Could you check a few things on this drawing? It's one solid part, dimensions in mm from its lowest x, y, z. A direction names the side the tool comes from. Give positions to 0.01 mm unless a question says otherwise; leave off trailing zeros. Loops run counter-clockwise (first coordinate to the right, second up) from the corner with the lowest first, then second, coordinate; pieces in that order, holes last. Notation, with made-up numbers: M 66,3 L 85,3 A37 cw 85,39 Z; hole C 36.5,30 d2. An arc over 180 degrees is marked long. Answer in a Markdown table with one row per item. Add a question column.
1. Which directions (+Z, -Z, +X, -X, +Y, -Y) give clear straight access to the entire face, cutting with the end or side of a thin tool? Please do the marked faces 1 and 2.
2. If we section it at A-A on x = 20: List the corners of the cut face in (y, z) for me.
3. I need wall thicknesses on line 1 along Z through (x, y) = (22.5, 36.5); line 2 along Y through (x, z) = (19.5, 6.5); line 3 along Y through (x, z) = (12, 4). Which ranges of each line are inside material? Lowest first, please. Write a range as from..to.
4. If we section it at C-C on z = 29: List the corners of the cut face in (x, y) for me, then the cut area to 3 significant figures.
5. I'm going to push flat-ended pins straight in: pin 1 Ø2 at (x, z) = (27.5, 11.5) entering from -Y; pin 2 Ø1.5 at (x, z) = (25.5, 8) entering from +Y; pin 3 Ø8 at (x, z) = (11.5, 21) entering from -Y. Where does each tip first touch, or does it pass through?
6. If we section it at D-D on x = 34.5: List the corners of the cut face in (y, z) for me.
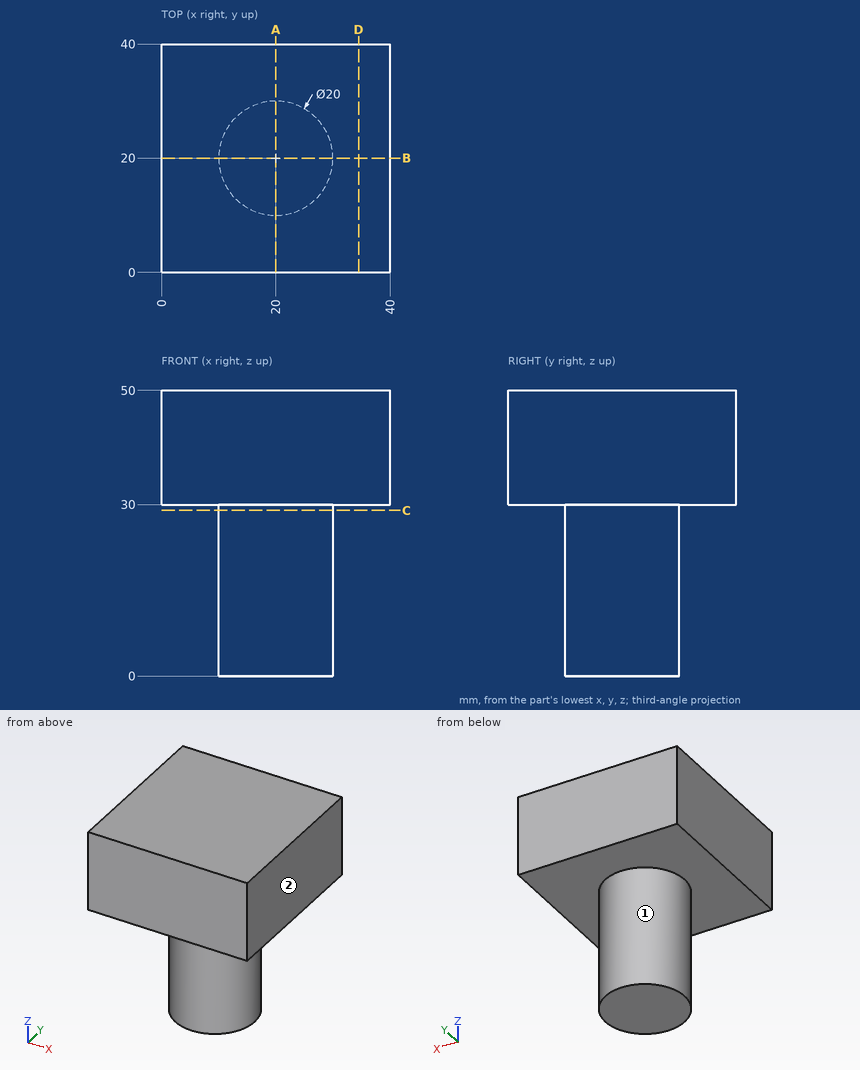
Results:
| question | item | result |
|---|---|---|
| 1 | face 1 | -Z |
| 1 | face 2 | +Z, -Z, +X, +Y, -Y |
| 2 | outline | M 0,30 L 10,30 L 10,0 L 30,0 L 30,30 L 40,30 L 40,50 L 0,50 Z |
| 3 | line 1 | 30..50 |
| 3 | line 2 | 10.01..29.99 |
| 3 | line 3 | 14..26 |
| 4 | outline | C 20,20 d20 |
| 4 | area | 314 mm2 |
| 5 | pin 1 | y = 12.4 |
| 5 | pin 2 | y = 28.8 |
| 5 | pin 3 | y = 11.07 |
| 6 | outline | M 0,30 L 40,30 L 40,50 L 0,50 Z |
